Work out the finished part from the listing and answer in its coordinate system (mm). Round coordinates to 2 decimals unless told otherwise and drop trailing zeros. Loops run counter-clockwise (first coordinate to the right, second up) from the corner with the lowest first, then second, coordinate; pieces in that order, holes last. Notation, with made-up numbers: M -29,-20.5 L 25,-20.5 A12 ccw 25,-11.5 Z; hole C 47,76 d9. An arc over 180 degrees is marked long. One line per item, written item: value.
```python
from build123d import *

# Parameters (mm, degrees)
SKIZZE1_W                       = 85
SKIZZE1_H                       = 30
AUFSATZ_LINEAR_AUSTRAGEN1_DEPTH = 3
SKIZZE2_R                       = 1.55
SCHNITT_LINEAR_AUSTRAGEN1_DEPTH = 4
SCHNITT_LINEAR_AUSTRAGEN2_DEPTH = 4
VERRUNDUNG1_R                   = 4


with BuildPart() as part:
    # Skizze1 → Aufsatz-Linear austragen1 (new body)
    with BuildSketch(Plane(origin=(0, 0, 0), x_dir=(0, 0, -1), z_dir=(1, 0, 0))):
        with Locations((42.5, 15)):
            Rectangle(SKIZZE1_W, SKIZZE1_H)
    extrude(amount=AUFSATZ_LINEAR_AUSTRAGEN1_DEPTH)

    # Skizze2 → Schnitt-Linear austragen1 (cut, through all)
    with BuildSketch(Plane(origin=(3, 0, 0), x_dir=(0, 0, -1), z_dir=(1, 0, 0))):
        with Locations((6, 22)):
            Circle(SKIZZE2_R)
        with Locations((27, 7)):
            Circle(SKIZZE2_R)
        with Locations((51.59187467, 7)):
            Circle(SKIZZE2_R)
        with Locations((76.183749339, 7)):
            Circle(SKIZZE2_R)
    extrude(amount=-SCHNITT_LINEAR_AUSTRAGEN1_DEPTH, mode=Mode.SUBTRACT)

    # Skizze3 → Schnitt-Linear austragen2 (cut, through all)
    with BuildSketch(Plane(origin=(3, 0, 0), x_dir=(0, 0, -1), z_dir=(1, 0, 0))):
        Polygon((0, 18.912292628), (26.47720968, 0), (0, 0), align=None)
    extrude(amount=-SCHNITT_LINEAR_AUSTRAGEN2_DEPTH, mode=Mode.SUBTRACT)

    # Verrundung1
    verrundung1_edges = [part.edges().sort_by_distance(p)[0] for p in [
        (1.5, 18.912292628, 0),
        (1.5, 30, 0),
        (1.5, 30, -85),
        (1.5, 0, -85),
    ]]
    fillet(verrundung1_edges, radius=VERRUNDUNG1_R)


solid = part.part
```
1) The mould has two halves that part along Z. Classify faces 1 (the face through (1.521, 6.406, -28.432)), 2 (the face through (1, 23, 0)), 3 (the face through (1.521, 28.859, -83.797)): +Z half, -Z half, draft (parallel to the pull), parting line (faces both ways), or undercut.
Check values:
face 1: undercut
face 2: +Z half
face 3: -Z half
2) Find section B-B (x = 2.1). Give the vertices of the cut face in (y, z).
Check values:
outline: M 0,-81 A4 ccw 4,-85 L 26,-85 A4 ccw 30,-81 L 30,-4 A4 ccw 26,0 L 20.97,0 A4 ccw 17.72,-1.68 L 0,-26.48 Z; hole C 7,-76.18 d3.1; hole C 7,-51.59 d3.1; hole C 7,-27 d3.1; hole C 22,-6 d3.1
3) This flat-tipped pin is pushed along its axis until it touches: pin 1 (3 mm diameter, centred on y = 7, z = -51.59, fed in from -X). Where does it stop, or does it pass through?
Check values:
pin 1: through
4) Find section C-C (y = 7). Give the vertices of the cut face in (x, z).
Check values:
outline: M 0,-85 L 3,-85 L 3,-77.73 L 0,-77.73 Z; M 0,-74.63 L 3,-74.63 L 3,-53.14 L 0,-53.14 Z; M 0,-50.04 L 3,-50.04 L 3,-28.55 L 0,-28.55 Z; M 0,-25.45 L 3,-25.45 L 3,-16.68 L 0,-16.68 Z
5) Find section D-D (z = -6). Give the vertices of the cut face in (x, y).
Check values:
outline: M 0,14.63 L 3,14.63 L 3,20.45 L 0,20.45 Z; M 0,23.55 L 3,23.55 L 3,30 L 0,30 Z
6) Find section A-A (y = 22). Give the vertices of the cut face in (x, z), then the cut area to 3 significant figures.
Check values:
outline: M 0,-85 L 3,-85 L 3,-7.55 L 0,-7.55 Z; M 0,-4.45 L 3,-4.45 L 3,0 L 0,0 Z
area: 246 mm2
7) Find the intervals of material crossed by probe 1 along Y at (x, z) = (1.3, -27); probe 2 along Z at (x, y) = (1.65, 8); probe 3 along Y at (x, z) = (1, -26), in increasing order. Write a range as from..to.
Check values:
probe 1: 0..5.45, 8.55..30
probe 2: -85..-77.37, -75..-52.78, -50.41..-28.18, -25.82..-15.28
probe 3: 0.34..5.82, 8.18..30
